Verification items for this drawing (mm, ordinates from the low corner). Coordinates: 2 decimals unless noted, no trailing zeros. Order: outer loops, then holes, each group sorted by start corner. A loop starts at its lowest first (then second) coordinate and runs counter-clockwise, first axis right, second up. Notation, with made-up numbers: M 75,-31 L 129,-31 A20 cw 129,-3 Z; hole C 11,26 d8. An arc over 180 degrees is marked long. One line per item, written item: value. Start each with the question number.
1) Go/stop test with a flat-tipped pin: P1, Ø1.5, axis at x = 56, y = 19, coming from the +Z side. Record where the tip stops, or that it passes through.
2) Sectioned sample at B-B, the plane x = 42.5. Enter the section's corners in (y, z) (1 decimal), then the cut area to 3 significant figures.
3) Thickness scan on L1, parallel to X at y = 3.5, z = 188.5 (1 decimal); L2, parallel to Z at x = 68.5, y = 43.5 (1 decimal); L3, parallel to Z at x = 45.5, y = 48 (1 decimal). Record the ranges inside material, lowest first. Write a range as from..to.
4) Sectioned sample at C-C, the plane z = 175.5. Enter the section's corners in (x, y) (1 decimal).
5) Sectioned sample at A-A, the plane y = 20. Enter the section's corners in (x, z), then the cut area to 3 significant figures.
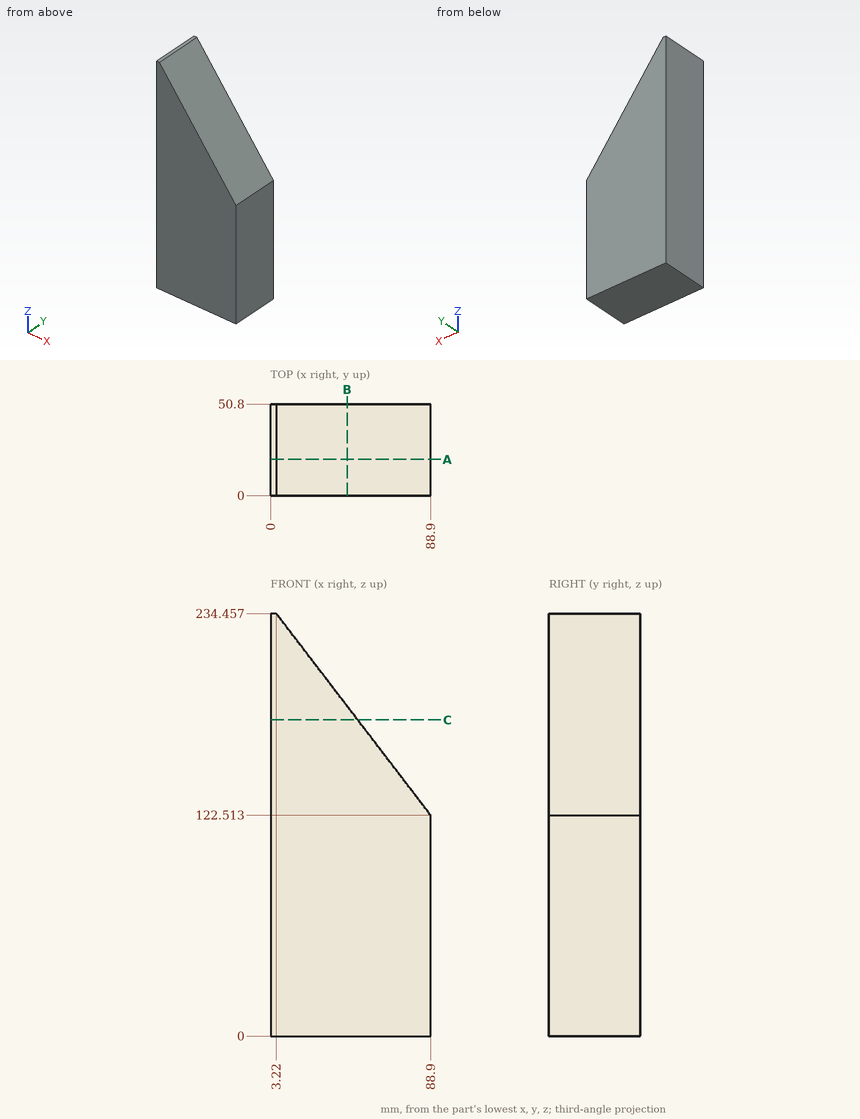
Final values:
1. P1: stops at z = 166.48
2. outline: M 0,0 L 50.8,0 L 50.8,183.1 L 0,183.1 Z
2. area: 9,300 mm^2
3. L1: x = 0..38.4
3. L2: z = 0..149.2
3. L3: z = 0..179.2
4. outline: M 0,0 L 48.3,0 L 48.3,50.8 L 0,50.8 Z
5. outline: M 0,0 L 88.9,0 L 88.9,122.51 L 3.22,234.46 L 0,234.46 Z
5. area: 16,000 mm^2
